Verification items for the finished model (mm, model axes). Round coordinates to 2 decimals unless told otherwise and drop trailing zeros. Write each loop counter-clockwise with the first axis right and the second up, starting at its lowest first coordinate (ties: lowest second). Pieces come first, ordered by that corner, then holes. Notation, with made-up numbers: M 23,9 L 59,9 A35 ccw 59,43 Z; hole C 76,55 d8. An arc over 180 degrees is marked long. Answer in a Markdown table with one row per item. Add a question column.
1. Material ranges on probe 1 along X at (y, z) = (-0.45, 0.05); probe 2 along Y at (x, z) = (3.5, -0.05); probe 3 along Y at (x, z) = (4.5, 0.35), recorded low to high.
2. Draft check along X on faces 1 (the cylindrical face through (4.2, -0.7, 0)), 2 (the cylindrical face through (0.28, 0.58, -0.18)), 3 (the flat face through (8, 0, 0)). Enter one of: pulls with the +X half, pulls with the -X half, needs draft (parallel to the pull), parting line crosses it, or undercut.
3. Sectioned sample at A-A on x = 3. Record the cut outline in (y, z).
4. Go/stop test with a flat-tipped pin: pin 1 Ø0.5 at (x, z) = (-0.5, -0.5) entering from +Y. Record where the tip stops, or that it passes through.
Autodesk Inventor part; units mm, degrees
ref_plane "IDS_WORKPLANE{1}" through (-1.0254, 0, 0) normal (1, 0, 0) x (0, 0, -1)
ref_plane "Work Plane2" through (8.25, 0, 0) normal (0, 0, -1) x (1, 0, 0)
ref_plane "YZ Plane" through (0, 0, 0) normal (1, 0, 0) x (0, 1, 0)
sketch "Sketch1" plane through (0, 0, 0) normal (0, 0, 1) x (1, 0, 0)
  line L0 (-1.0254, 0) -> (8, 0)
  line L1 (8, 0) -> (8, 0.7)
  line L2 (8, 0.7) -> (0.75, 0.7)
  line L3 (0.75, 0.7) -> (0.566, 0.608)
  line L4 (0.566, 0.608) -> (0, 0.608)
  line L5 (0, 0.608) -> (0, 1.3)
  line L6 (-4.8605, 0) -> (21.908, 0)
  line L7 (0, -0.26) -> (0, 1.5602)
  line L8 (0, 1.3) -> (-0.9811, 1.2998)
  arc A0 (-0.9811, 1.2998) -> (-1.0254, 0) centre (18.0839, 0) ccw
  dimension "d0" = 8
  dimension "d1" = 7.25
  dimension "d2" = 0.184
  dimension "d3" = 1.0254
  dimension "d4" = 1.4
  dimension "d5" = 1.216
  dimension "d9" = 2.6
  dimension "d10" = 0.01
  dimension "d15" = 19.1093
revolve "Body" add sketch "Sketch1" angle 360 about axis through (-1.0254, 0, 0) along (1, 0, 0)
fillet "Fillet1" radius 0.9 1 edges at (-0.9811, -1.2998, 0)
ref_plane "IDS_WORKPLANE{1}" through (-1.0254, 0, 0) normal (1, 0, 0) x (0, 0, -1)
sketch "Sketch2" plane through (-1.0254, 0, 0) normal (1, 0, 0) x (0, 0, -1)
  line L0 (0, -1.82) -> (0, 1.82)
  line L1 (1.82, 0) -> (-1.82, 0)
  line L2 (-1.3, 0.16) -> (1.3, 0.16)
  line L3 (1.3, 0.16) -> (1.3, -0.16)
  line L4 (1.3, -0.16) -> (-1.3, -0.16)
  line L5 (-1.3, -0.16) -> (-1.3, 0.16)
  line L6 (0, 0.16) -> (0, -0.16) construction
  line L7 (-1.3, 0) -> (1.3, 0) construction
  circle A0 centre (0, 0) radius 1.3
  dimension "d17" = 0.32
extrude "Slot" cut sketch "Sketch2" along normal blind 0.6 contours L4 A0 L1 L0 | L0 L1 A0 L4 | L4 L5 A0 | A0 L3 L4 | L1 A0 L2 L0 | L0 L2 A0 L1 | L5 L2 A0 | A0 L2 L3
thread "Thread"
chamfer "Chamfer1" distance 0.184 distance2 0.1841 1 edges at (8, -0.7, 0) measured on face at (8, 0.4839, -0.1193)
ref_plane "Work Plane2" through (8.25, 0, 0) normal (0, 0, -1) x (1, 0, 0)
equation "\"d17\" = SBR"
equation "\"d18\" = STI"
equation "\"d20\" = RR"
equation "\"d11\" = GEL"
equation "\"d13\" = -0.5 * SPD + 0.5 * GD"
equation "\"d0\" = NLG"
equation "\"d1\" = GEL"
equation "\"d2\" = GAL"
equation "\"d3\" = KOH"
equation "\"d4\" = GD"
equation "\"d5\" = BDM"
equation "\"d9\" = KOD"
equation "\"d10\" = KEWI"
equation "\"GD\" = NND"
equation "\"NLG\" = 8"
equation "\"GEL\" = 7.25"
equation "\"KOD\" = 2.6"
equation "\"KOH\" = 1.02539"
equation "\"GAL\" = 0.61345 * PTC"
equation "\"SPD\" = NND - 1.2269 * PTC"
equation "\"BDM\" = 1.216"
equation "\"GUL\" = 0.61345 * PTC"
equation "\"RR\" = 0.9"
equation "\"SBR\" = 0.32"
equation "\"STI\" = 0.6"
equation "\"KEWI\" = 0.01deg"
equation "\"KR\" = 1.6"
equation "\"d16\" = -KOH"
equation "\"PTC\" = 0.3"
equation "\"THREADDIA\" = 1.4"
equation "\"TOA\" = 30deg"
equation "\"NND\" = 1.4"
equation "\"ORI\" = 0.9"
equation "\"GD1\" = THREADDIA - 1.2269 * PTC"
properties part number "CNS 9671 - M1,4 x 8" material "Steel, Mild"
Geometry check:
| question | item | result |
|---|---|---|
| 1 | probe 1 | x = -1.02 to 8 |
| 1 | probe 2 | y = -0.7 to 0.7 |
| 1 | probe 3 | y = -0.61 to 0.61 |
| 2 | face 1 | needs draft |
| 2 | face 2 | undercut |
| 2 | face 3 | pulls with the +X half |
| 3 | outline | C 0,0 d1.4 |
| 4 | pin 1 | stops at y = 1.24 |
